Here's how the part is built. I have some questions about the finished solid (model axes, mm). A direction names the side the tool comes from. Give positions to 0.01 mm unless a question says otherwise; leave off trailing zeros. Loops run counter-clockwise (first coordinate to the right, second up) from the corner with the lowest first, then second, coordinate; pieces in that order, holes last. Notation, with made-up numbers: (-34, -0.5) - (21, -0.5) arc R27 cw to (21, 24.5) - close; hole circle Ø9 at (29, -34). An arc over 180 degrees is marked (long way). Use one line per item in the form item = value.
from build123d import *

# Parameters (mm, degrees)
F0_W     = 93.98
F0_H     = 82.55
F1_DEPTH = 2.54
F2_W     = 8.89
F2_H     = 8.89
F3_DEPTH = 16.51
F6_D     = 1.905
F9_D     = 1.905
F9_DEPTH = 12.7


with BuildPart() as f1:
    # F0 (on Right) → F1 (new body)
    with BuildSketch(Plane.YZ):
        with Locations((7.112141, -1.921732)):
            Rectangle(F0_W, F0_H)
    extrude(amount=F1_DEPTH)

    # F2 (on face) → F3 (join)
    with BuildSketch(Plane(origin=(0, 0, 0), x_dir=(0, -1, 0), z_dir=(-1, 0, 0))):
        with Locations((-47.117141, 34.908268)):
            Rectangle(F2_W, F2_H)
        with Locations((32.892859, 34.908268)):
            Rectangle(F2_W, F2_H)
        with Locations((32.892859, -36.211732)):
            Rectangle(F2_W, F2_H)
        with Locations((-47.117141, -36.211732)):
            Rectangle(F2_W, F2_H)
    extrude(amount=F3_DEPTH)

    # F6 (through all)
    with Locations(Plane.XZ.offset(37.337859)):
        with Locations((-11.43, -36.211732), (-11.43, 34.908268)):
            Hole(F6_D / 2)

    # F9
    with Locations(Plane(origin=(0, 0, -40.656732), x_dir=(1, 0, 0), z_dir=(0, 0, -1))):
        with Locations((-4.445, -47.117141), (-4.445, 32.892859)):
            Hole(F9_D / 2, depth=F9_DEPTH)


solid = f1.part
(1) For faces 1 (the flat face through (-8, -28.448, 35)), 2 (the flat face through (-8, -33, -40.657)), 3 (the flat face through (-8, 47, 30.463)), which set-ups out of +Z, -Z, +X, -X, +Y, -Y let a thin tool reach every point of the face, with its end or its side?
Geometry says:
face_1 = +Z, -Z, -X
face_2 = -Z, -X, +Y, -Y
face_3 = -X, +Y, -Y
(2) For P1, Ø7, axis at x = -11.5, y = 45.5, coming from the -Z side; P2, Ø4.5, axis at x = -4.5, z = -37.5, coming from the -Y side; P3, Ø1.1, axis at x = -11.43, z = 34.91, coming from the -Y side; P4, Ø12, axis at y = 28.5, z = -23.5, coming from the -X side, each with a flat end and sliding along its axis, tell me the tip position at first contact or that it passes through.
Geometry says:
P1 = -40.66
P2 = -37.34
P3 = through
P4 = 0
(3) If we section it at B-B (y = -12): List the corners of the cut face in (x, z) for me.
Geometry says:
outline = (0, -43.2) - (2.54, -43.2) - (2.54, 39.35) - (0, 39.35) - close
(4) If we section it at A-A (z = 9.5): List the corners of the cut face in (x, y) for me, plus the area to 3 significant figures.
Geometry says:
outline = (0, -39.88) - (2.54, -39.88) - (2.54, 54.1) - (0, 54.1) - close
area = 239 mm²
(5) Thinking about a two-plate mould opening in Y: for faces 4 (the flat face through (-16.51, -33, 35)), 5 (the flat face through (-8, 51.562, -36)), 6 (the flat face through (-8, -37.338, -36)), 7 (the flat face through (-8, -28.448, -36)), which applies, pulls with the +Y half, pulls with the -Y half, needs draft (parallel to the pull), parting line crosses it, or undercut?
Geometry says:
face_4 = needs draft
face_5 = pulls with the +Y half
face_6 = pulls with the -Y half
face_7 = undercut
(6) If I drill on probe 1 along Z at (x, y) = (-11.43, -32.5); probe 2 along Y at (x, z) = (-10.5, 32); probe 3 along X at (y, z) = (30, -38), over which ranges is the centre line in solid material (lowest first)?
Geometry says:
probe_1 = -40.66 to -37.16, -35.26 to -31.77, 30.46 to 33.96, 35.86 to 39.35
probe_2 = -37.34 to -28.45, 42.67 to 51.56
probe_3 = 0 to 2.54
